Could you check a few things on this drawing? It's one solid part, dimensions in mm from its lowest x, y, z. A direction names the side the tool comes from. Give positions to 0.01 mm unless a question says otherwise; leave off trailing zeros. Order: outer loops, then holes, each group sorted by start corner. A loop starts at its lowest first (then second) coordinate and runs counter-clockwise, first axis right, second up.
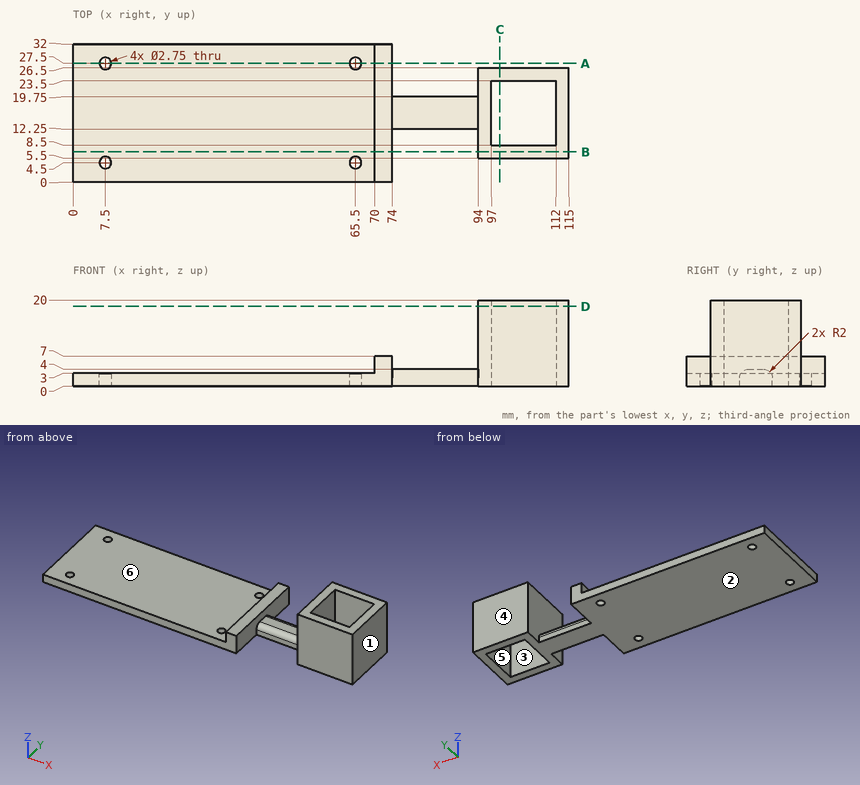
Item 1: For pin 1 (1 mm diameter, centred on x = 39.5, y = 9, fed in from -Z); pin 2 (3.5 mm diameter, centred on x = 65.5, y = 27.5, fed in from +Z); pin 3 (1 mm diameter, centred on x = 79.5, z = 1, fed in from +Y); pin 4 (12 mm diameter, centred on x = 107.5, z = 7.5, fed in from -Y), each with a flat end and sliding along its axis, tell me the tip position at first contact or that it passes through.
Findings:
pin 1: stops at z = 0
pin 2: stops at z = 3
pin 3: stops at y = 19.75
pin 4: stops at y = 5.5
Item 2: Imagine slicing it at C-C on x = 99. List the corners of the cut face in (y, z) for me, then the cut area to 3 significant figures.
Findings:
outline: (5.5, 0) - (8.5, 0) - (8.5, 20) - (5.5, 20) - close; (23.5, 0) - (26.5, 0) - (26.5, 20) - (23.5, 20) - close
area: 120 mm2
Item 3: Please list where these lines run through material, in increasing order: line 1 along X through (y, z) = (21.5, 1); line 2 along Y through (x, z) = (65.5, 1.8) (3 decimals); line 3 along X through (y, z) = (15, 10.75).
Findings:
line 1: x = 0 to 74, 94 to 97, 112 to 115
line 2: y = 0 to 3.125, 5.875 to 26.125, 28.875 to 32
line 3: x = 94 to 97, 112 to 115
Item 4: Imagine slicing it at B-B on y = 7. List the corners of the cut face in (x, z) for me, then the cut area to 3 significant figures.
Findings:
outline: (0, 0) - (74, 0) - (74, 7) - (70, 7) - (70, 3) - (0, 3) - close; (94, 0) - (115, 0) - (115, 20) - (94, 20) - close
area: 658 mm2
Item 5: Imagine slicing it at D-D on z = 18.5. List the corners of the cut face in (x, y) for me, then the cut area to 3 significant figures.
Findings:
outline: (94, 5.5) - (115, 5.5) - (115, 26.5) - (94, 26.5) - close; hole (97, 8.5) - (112, 8.5) - (112, 23.5) - (97, 23.5) - close
area: 216 mm2
Item 6: For the marked faces 4, 5 and 6, which set-ups out of +Z, -Z, +X, -X, +Y, -Y let a thin tool reach every point of the face, with its end or its side?
Findings:
face 4: +Z, -Z, +X, +Y
face 5: +Z, -Z
face 6: +Z, -X, +Y, -Y
Item 7: We'd pull the mould along X, two halves only. Please class the marked faces 1, 2 and 3: +X half, -X half, draft (parallel to the pull), parting line (faces both ways), or undercut.
Findings:
face 1: +X half
face 2: draft
face 3: undercut
Item 8: Imagine slicing it at A-A on y = 27.5. List the corners of the cut face in (x, z) for me (3 decimals), then the cut area to 4 significant figures.
Findings:
outline: (0, 0) - (6.125, 0) - (6.125, 3) - (0, 3) - close; (8.875, 0) - (64.125, 0) - (64.125, 3) - (8.875, 3) - close; (66.875, 0) - (74, 0) - (74, 7) - (70, 7) - (70, 3) - (66.875, 3) - close
area: 221.5 mm2
